Read the model definition and answer for the solid it produces. Units are mm, in the model's axes. Give positions to 0.01 mm unless a question says otherwise; leave off trailing zeros. Order: outer loops, then holes, each group sorted by start corner. A loop starts at its lowest first (then second) coordinate and runs counter-clockwise, first axis right, second up. Notation, with made-up numbers: (31.5, -36) - (36.5, -36) arc R21 cw to (36.5, 2) - close; hole circle Ø8 at (-15, 19). An arc over 180 degrees is marked (long way). Use a Markdown table: item, result. Add a question column.
1. Consider L1, parallel to X at y = -300, z = 28.85; L2, parallel to Y at x = 8.5, z = 27.15; L3, parallel to Y at x = 16.5, z = 27.55. Determine where each line is inside the solid, lowest interval first.
2. A cutting plane is placed at A-A on y = -208. Determine the outline of the cut face in (x, z).
3. A cutting plane is placed at B-B on z = 26.25. Determine the outline of the cut face in (x, y), and give its area (3 significant figures).
4. Flat-ended cylindrical pins translate along their axes: P1, Ø1, axis at y = -197.5, z = 25.5, coming from the +X side; P2, Ø1.5, axis at y = -102, z = 28.5, coming from the +X side; P3, Ø1, axis at y = -82.5, z = 28.5, coming from the +X side; P4, Ø4.5, axis at x = -70, y = -250, coming from the +Z side. Find the tip coordinate at first contact, or state that the pin passes through.
5. A cutting plane is placed at C-C on x = 0. Determine the outline of the cut face in (y, z), and give its area (3 significant figures).
6. A cutting plane is placed at D-D on y = -7.5. Determine the outline of the cut face in (x, z).
```python
from build123d import *

# Parameters (mm, degrees)
SKETCH_1_R                = 20
SKETCH_1_R_2              = 11.1
EXTRUDE_1_DEPTH           = 60
EXTRUDE_2_DEPTH           = 30
SKETCH_4_R                = 11
EXTRUDE_3_DEPTH           = 5
SKETCH_8_R                = 11.1
CUT_EXTRUDE_1_DEPTH       = 100
FILLET_4_R                = 20
EXTRUDE_START             = -30
SKETCH_18_R               = 35
EXTRUDE_4_DEPTH           = 5
EXTRUDE_START_2           = -25
SKETCH_19_R               = 35
EXTRUDE_5_DEPTH           = 5
FILLET_5_R                = 10
CUT_EXTRUDE_9_DEPTH       = 388.169213652
CUT_EXTRUDE_9_DEPTH_BACK  = 388.169213652
SKETCH_21_R               = 2.6
CUT_EXTRUDE_10_DEPTH      = 409.372938359
CUT_EXTRUDE_10_DEPTH_BACK = 409.372938359
SKETCH_22_W               = 30
SKETCH_22_H               = 469.737304999
SKETCH_22_W_2             = 35
SKETCH_22_H_2             = 431.087956996


with BuildPart() as part:
    # 草图1 → 凸台-拉伸1 (new body)
    with BuildSketch(Plane.XY):
        Circle(SKETCH_1_R)
        Circle(SKETCH_1_R_2, mode=Mode.SUBTRACT)
    extrude(amount=EXTRUDE_1_DEPTH)

    # 草图2 → 凸台-拉伸2 (add, symmetric)
    with BuildSketch(Plane.XY.offset(30)):
        with BuildLine():
            Line((-14.142135624, 14.142135624), (-90, -61.715728753))
            Line((-90, -61.715728753), (-90, -320))
            Line((-90, -320), (-50, -320))
            Line((-50, -320), (-50, -78.284271247))
            Line((-50, -78.284271247), (14.142135624, -14.142135624))
            ThreePointArc((14.142135624, -14.142135624), (-14.142135624, -14.142135624), (-14.142135624, 14.142135624))
        make_face()
    extrude(amount=EXTRUDE_2_DEPTH, both=True)

    # 草图4 → 凸台-拉伸3 (add)
    with BuildSketch(Plane.XY.offset(60)):
        with BuildLine():
            Line((-90, -290), (-50, -290))
            Line((-50, -290), (-50, -350))
            ThreePointArc((-50, -350), (-70, -370), (-90, -350))
            Line((-90, -350), (-90, -290))
        make_face()
        with Locations((-70, -350)):
            Circle(SKETCH_4_R, mode=Mode.SUBTRACT)
    extrude_3 = extrude(amount=EXTRUDE_3_DEPTH)

    # 镜向1: 凸台-拉伸3 across plane
    add(extrude_3.mirror(Plane.XY.offset(30)))

    # 草图8 → 切除-拉伸1 (cut)
    with BuildSketch(Plane.XY.offset(60)):
        with Locations((-35.355339059, -35.355339059)):
            Circle(SKETCH_8_R)
    extrude(amount=-CUT_EXTRUDE_1_DEPTH, mode=Mode.SUBTRACT)

    # 圆角4
    fillet_4_edges = [part.edges().sort_by_distance(p)[0] for p in [
        (-50, -78.284271247, 30),
        (-90, -61.715728753, 30),
    ]]
    fillet(fillet_4_edges, radius=FILLET_4_R)

    # 草图18 → 凸台-拉伸4 (add)
    with BuildSketch(Plane.XY.offset(60).offset(EXTRUDE_START)):
        with BuildLine():
            ThreePointArc((16.783988507, -10.876475983), (15.54903282, -12.578854413), (14.142135624, -14.142135624))
            Line((14.142135624, -14.142135624), (-44.142135624, -72.426406871))
            ThreePointArc((-44.142135624, -72.426406871), (-48.47759065, -78.914873848), (-50, -86.568542495))
            Line((-50, -86.568542495), (-50, -129.282056212))
            Line((-50, -129.282056212), (24.135744866, -129.282056212))
            ThreePointArc((24.135744866, -129.282056212), (66.634203362, -100.885494101), (56.662656801, -50.755144277))
            Line((56.662656801, -50.755144277), (16.783988507, -10.876475983))
        make_face()
        with Locations((24.135744866, -83.282056212)):
            Circle(SKETCH_18_R, mode=Mode.SUBTRACT)
    extrude(amount=EXTRUDE_4_DEPTH)

    # 草图19 → 凸台-拉伸5 (add)
    with BuildSketch(Plane(origin=(0, 0, 0), x_dir=(-1, 0, 0), z_dir=(0, 0, -1)).offset(EXTRUDE_START_2)):
        with BuildLine():
            Line((50, -135.340123781), (50, -227.340123781))
            Line((50, -227.340123781), (-4.524131353, -227.340123781))
            ThreePointArc((-4.524131353, -227.340123781), (-50.524131353, -181.340123781), (-4.524131353, -135.340123781))
            Line((-4.524131353, -135.340123781), (50, -135.340123781))
        make_face()
        with Locations((-4.524131353, -181.340123781)):
            Circle(SKETCH_19_R, mode=Mode.SUBTRACT)
    extrude(amount=-EXTRUDE_5_DEPTH)

    # 圆角5
    # the kernel refuses this fillet: 10 mm, written as the material it adds along each edge
    with BuildSketch(Plane(origin=(-50, -227.340123781, 25), x_dir=(0, -1, 0), z_dir=(0, 0, 1)), Plane(origin=(-50, -129.282056212, 30), x_dir=(0, -1, 0), z_dir=(0, 0, 1))) as fillet_5_piece_1:
        with BuildLine():
            CenterArc((FILLET_5_R, FILLET_5_R), FILLET_5_R, 180, 90)
            Line((0, FILLET_5_R), (0, 0))
            Line((0, 0), (FILLET_5_R, 0))
        make_face()
    extrude(amount=5)

    # 草图21 → 切除-拉伸9 (cut, two sides: drawn at the far end of the back side and taken through both)
    with BuildSketch(Plane.XY.offset(65).offset(-CUT_EXTRUDE_9_DEPTH_BACK)):
        with Locations((-70, -75)):
            Circle(SKETCH_21_R)
        with Locations((-70, -250)):
            Circle(SKETCH_21_R)
        with Locations((-58, -300)):
            Circle(SKETCH_21_R)
        with Locations((-82, -300)):
            Circle(SKETCH_21_R)
    extrude(amount=CUT_EXTRUDE_9_DEPTH + CUT_EXTRUDE_9_DEPTH_BACK, mode=Mode.SUBTRACT)

    # 草图22 → 切除-拉伸10 (cut, two sides: drawn at the far end of the back side and taken through both)
    with BuildSketch(Plane.ZY.offset(90).offset(-CUT_EXTRUDE_10_DEPTH_BACK)):
        with Locations((10, -169.950732915)):
            Rectangle(SKETCH_22_W, SKETCH_22_H)
        with Locations((47.5, -154.456021502)):
            Rectangle(SKETCH_22_W_2, SKETCH_22_H_2)
    extrude(amount=CUT_EXTRUDE_10_DEPTH + CUT_EXTRUDE_10_DEPTH_BACK, mode=Mode.SUBTRACT)


solid = part.part
```
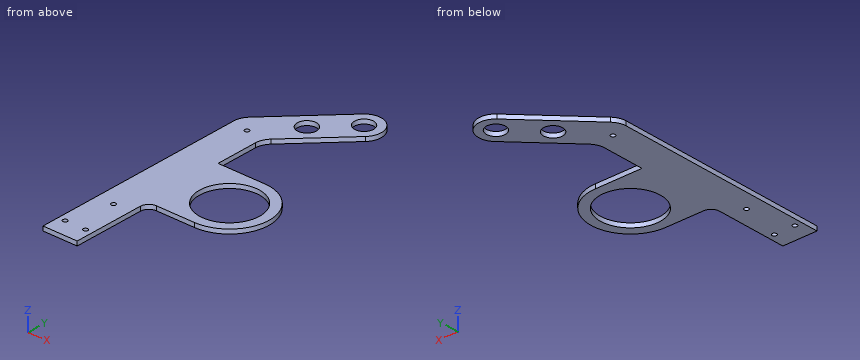
Output values:
| question | item | result |
|---|---|---|
| 1 | L1 | -90 to -84.6, -79.4 to -60.6, -55.4 to -50 |
| 1 | L2 | -227.17 to -216.11, -146.57 to -135.51, -19.78 to -7.14, 7.14 to 18.1 |
| 1 | L3 | -225.75 to -214.23, -148.45 to -136.93, -11.3 to 11.3 |
| 2 | outline | (-90, 25) - (-18.15, 25) - (-18.15, 30) - (-90, 30) - close; (27.2, 25) - (42.01, 25) - (42.01, 30) - (27.2, 30) - close |
| 3 | outline | (-90, -320) - (-50, -320) - (-50, -237.34) arc R10 cw to (-40, -227.34) - (4.52, -227.34) arc R46 ccw to (4.52, -135.34) - (-50, -135.34) - (-50, -86.57) arc R20 cw to (-44.14, -72.43) - (14.14, -14.14) arc R20 ccw to (-14.14, 14.14) - (-84.14, -55.86) arc R20 ccw to (-90, -70) - close; hole circle Ø5.2 at (-82, -300); hole circle Ø5.2 at (-70, -250); hole circle Ø5.2 at (-70, -75); hole circle Ø5.2 at (-58, -300); hole circle Ø22.2 at (-35.36, -35.36); hole circle Ø70 at (4.52, -181.34); hole circle Ø22.2 at (0, 0) |
| 3 | area | 18,200 mm² |
| 4 | P1 | x = 47.78 |
| 4 | P2 | x = -50 |
| 4 | P3 | x = -49.47 |
| 4 | P4 | through |
| 5 | outline | (-227.34, 25) - (-216.05, 25) - (-216.05, 30) - (-227.34, 30) - close; (-146.63, 25) - (-135.34, 25) - (-135.34, 30) - (-146.63, 30) - close; (-28.28, 25) - (-11.1, 25) - (-11.1, 30) - (-28.28, 30) - close; (11.1, 25) - (20, 25) - (20, 30) - (11.1, 30) - close |
| 5 | area | 243 mm² |
| 6 | outline | (-35.78, 25) - (-8.18, 25) - (-8.18, 30) - (-35.78, 30) - close; (8.18, 25) - (18.54, 25) - (18.54, 30) - (8.18, 30) - close |
